Study the drawing (mm; zero at the part's minimum x, y, z) and answer. Give positions to 0.01 mm unless a question says otherwise; leave off trailing zeros. Order: outer loops, then holes, each group sorted by start corner. A loop starts at its lowest first (then second) coordinate and runs counter-clockwise, first axis right, second up. Notation, with made-up numbers: (6.25, 36) - (48.25, 36) arc R11 ccw to (48.25, 53) - close; hole circle Ø6 at (83, 60.25). An arc over 180 degrees is marked (long way). Use CSV: the item, a comma, the result in double quotes.
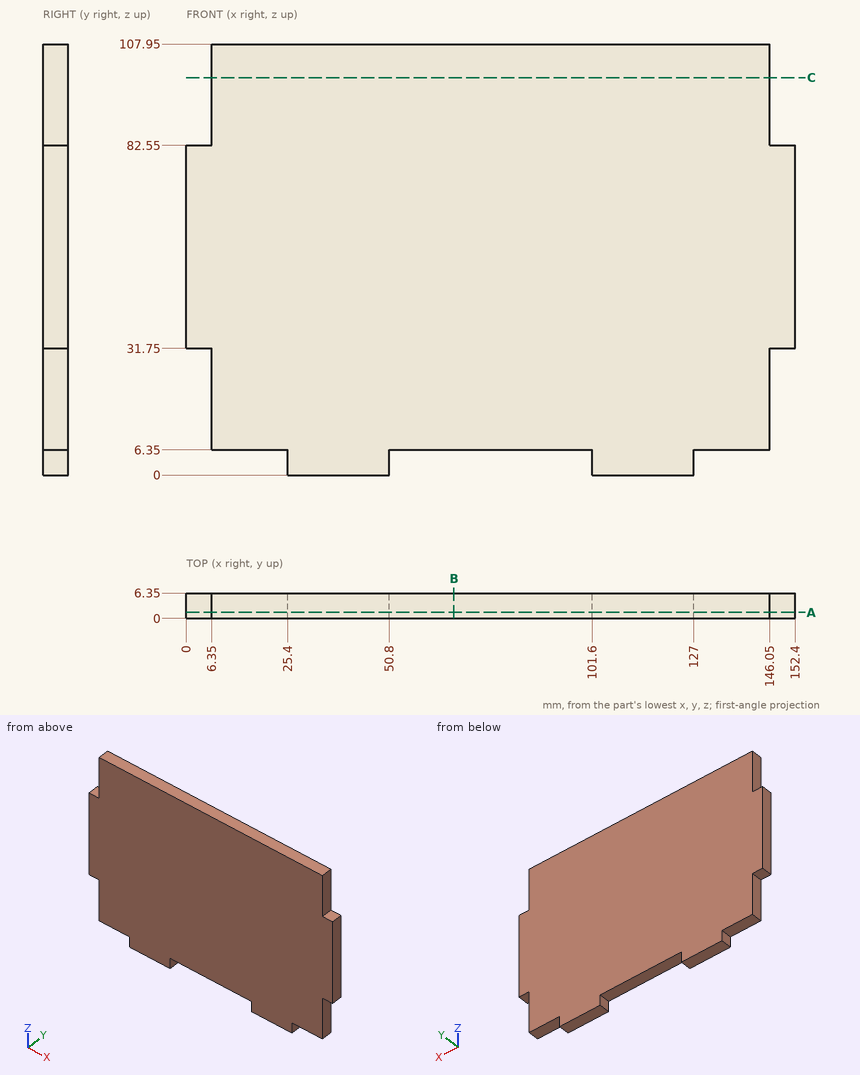
Item 1: The part is cut by section B-B (x = 67). Give the vertices of the cut face in (y, z).
Taken from the geometry:
outline,"(0, 6.35) - (6.35, 6.35) - (6.35, 107.95) - (0, 107.95) - close"
Item 2: The part is cut by section C-C (z = 99.5). Give the vertices of the cut face in (x, y), and give its area (3 significant figures).
Taken from the geometry:
outline,"(6.35, 0) - (146.05, 0) - (146.05, 6.35) - (6.35, 6.35) - close"
area,"887 mm^2"
Item 3: The part is cut by section A-A (y = 1.5). Give the vertices of the cut face in (x, z), and give its area (3 significant figures).
Taken from the geometry:
outline,"(0, 31.75) - (6.35, 31.75) - (6.35, 6.35) - (25.4, 6.35) - (25.4, 0) - (50.8, 0) - (50.8, 6.35) - (101.6, 6.35) - (101.6, 0) - (127, 0) - (127, 6.35) - (146.05, 6.35) - (146.05, 31.75) - (152.4, 31.75) - (152.4, 82.55) - (146.05, 82.55) - (146.05, 107.95) - (6.35, 107.95) - (6.35, 82.55) - (0, 82.55) - close"
area,"15,200 mm^2"
Item 4: Each of these flat-tipped pins is pushed along its axis until it touches: pin 1 (3 mm diameter, centred on x = 2, y = 3.5, fed in from -Z); pin 2 (3 mm diameter, centred on y = 4.5, z = 20, fed in from -X); pin 3 (1.9 mm diameter, centred on x = 75, y = 4, fed in from -Z). Where does it stop, or does it pass through?
Taken from the geometry:
pin 1,"z = 31.75"
pin 2,"x = 6.35"
pin 3,"z = 6.35"
Item 5: Find the intervals of material crossed by line 1 along X through (y, z) = (1, 6); line 2 along Z through (x, y) = (76, 4.75); line 3 along X through (y, z) = (4, 103), in increasing order.
Taken from the geometry:
line 1,"25.4 to 50.8, 101.6 to 127"
line 2,"6.35 to 107.95"
line 3,"6.35 to 146.05"
